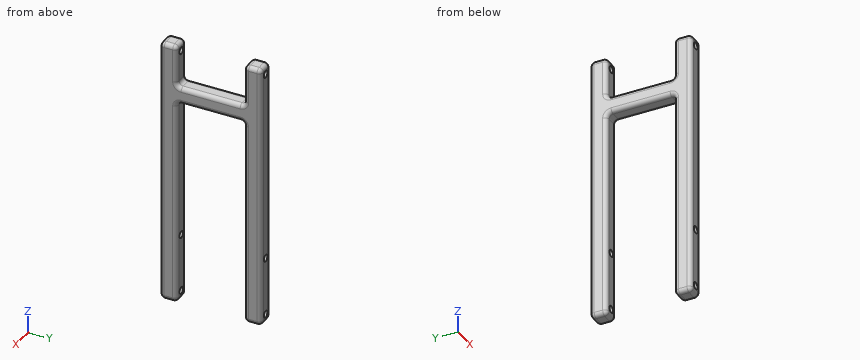
Autodesk Inventor part; units mm, degrees
ref_plane "YZ Plane" through (0, 0, 0) normal (1, 0, 0) x (0, 1, 0)
ref_plane "XZ Plane" through (0, 0, 0) normal (0, 1, 0) x (-1, 0, 0)
ref_plane "XY Plane" through (0, 0, 0) normal (0, 0, 1) x (1, 0, 0)
sketch "Sketch1" plane through (0, 0, 0) normal (0, 1, 0) x (-1, 0, 0)
  line L0 (0, 0) -> (12.7, 0)
  line L1 (12.7, 0) -> (12.7, 203.2)
  line L2 (12.7, 203.2) -> (0, 203.2)
  line L3 (0, 203.2) -> (0, 0)
  circle A0 centre (6.35, 6.35) radius 2.5797
  circle A1 centre (6.35, 196.85) radius 2.5797
  circle A2 centre (6.35, 50.8) radius 2.5797
  dimension "d0" = 12.7
  dimension "d1" = 203.2
  dimension "d2" = 6.35
  dimension "d3" = 6.35
  dimension "d4" = 5.1594
  dimension "d5" = 6.35
  dimension "d6" = 5.1594
  dimension "d7" = 6.35
  dimension "d19" = 5.1594
  dimension "d20" = 6.35
  dimension "d21" = 50.8
extrude "Extrusion1" add sketch "Sketch1" along normal blind 76.2
sketch "Sketch2" plane through (0, 0, 203.2) normal (1, 0, 0) x (0, 0, -1)
  line L0 (203.2, 76.2) -> (0, 76.2)
  line L1 (0, 76.2) -> (31.75, 76.2)
  line L2 (31.75, 76.2) -> (31.75, 0)
  line L3 (31.75, 0) -> (0, 0)
  line L4 (0, 0) -> (0, 76.2)
  line L5 (203.2, 76.2) -> (177.8, 76.2)
  line L6 (177.8, 76.2) -> (177.8, 0)
  line L7 (177.8, 0) -> (203.2, 0)
  line L8 (203.2, 0) -> (203.2, 76.2)
  line L9 (203.2, 0) -> (203.2, 76.2)
  line L10 (203.2, 63.5) -> (0, 63.5)
  line L11 (0, 63.5) -> (0, 12.7)
  line L12 (0, 12.7) -> (203.2, 12.7)
  line L13 (203.2, 12.7) -> (203.2, 63.5)
  line L14 (0, 0) -> (203.2, 0)
  line L15 (31.75, 63.5) -> (44.45, 63.5)
  line L16 (44.45, 63.5) -> (44.45, 12.7)
  line L17 (44.45, 12.7) -> (31.75, 12.7)
  line L18 (31.75, 12.7) -> (31.75, 63.5)
  line L19 (177.8, 63.5) -> (165.1, 63.5)
  line L20 (165.1, 12.7) -> (177.8, 12.7)
  line L21 (177.8, 12.7) -> (177.8, 63.5)
  line L22 (139.7, 63.5) -> (139.7, 12.7)
  line L23 (139.7, 63.5) -> (127, 63.5)
  line L24 (127, 63.5) -> (127, 12.7)
  line L25 (127, 12.7) -> (139.7, 12.7)
  line L26 (139.7, 12.7) -> (139.7, 63.5)
  point P0 (177.8, 12.7)
  point P1 (184.15, 63.5)
  point P2 (0, 12.7)
  point P3 (31.75, 12.7)
  point P4 (19.05, 63.5)
  point P5 (0, 63.5)
  point P6 (44.45, 63.5)
  point P7 (31.75, 12.7)
  dimension "d10" = 31.75
  dimension "d12" = 25.4
  dimension "d13" = 76.2
  dimension "d14" = 203.2
  dimension "d15" = 50.8
  dimension "d16" = 12.7
  dimension "d22" = 12.7
  dimension "d24" = 63.5
  dimension "d25" = 12.7
extrude "Extrusion2" cut sketch "Sketch2" against normal blind 12.7 contours L8 L12 L6 L10 | L6 L12 L22 L10 | L2 L12 L4 L10 | L10 L24 L12 L16 | L22 L12 L24 L10
fillet "Fillet1" radius 3.175 36 edges at (0, 38.1, 158.75) (0, 38.1, 171.45) (-12.7, 38.1, 171.45) (-12.7, 38.1, 158.75) (0, 63.5, 79.375) (0, 76.2, 101.6) (-12.7, 76.2, 101.6) (-12.7, 63.5, 79.375) (0, 63.5, 187.325) (-12.7, 63.5, 187.325) (-6.35, 63.5, 158.75) (-6.35, 63.5, 171.45) (-12.7, 12.7, 79.375) (0, 12.7, 79.375) (-12.7, 0, 101.6) (0, 0, 101.6) (0, 12.7, 187.325) (-12.7, 12.7, 187.325) (-6.35, 12.7, 171.45) (-6.35, 12.7, 158.75) (-6.35, 12.7, 203.2) (0, 6.35, 203.2) (-6.35, 0, 203.2) (-12.7, 6.35, 203.2) (0, 6.35, 0) (-6.35, 0, 0) (-12.7, 6.35, 0) (-6.35, 12.7, 0) (-6.35, 76.2, 0) (0, 69.85, 0) (-6.35, 63.5, 0) (-12.7, 69.85, 0) (0, 69.85, 203.2) (-6.35, 63.5, 203.2) (-12.7, 69.85, 203.2) (-6.35, 76.2, 203.2)
properties part number "inner swing"
Geometry: final body of the model. Coordinates: model frame, mm. Give positions to 0.01 mm unless a question says otherwise; leave off trailing zeros. Write each loop counter-clockwise with the first axis right and the second up, starting at its lowest first coordinate (ties: lowest second). Pieces come first, ordered by that corner, then holes. Notation, with made-up numbers: M -37,-15 L -12,-15 A33 cw -12,24 Z; hole C 0,-31.75 d6. An arc over 180 degrees is marked long. Answer in a Markdown table with one row per item. Add a question column.
(1) First-contact query: pin 1 (5 mm diameter, centred on x = -10.5, y = 29, fed in from -Z); pin 2 (6 mm diameter, centred on x = -4, y = 60, fed in from +Z); pin 3 (3 mm diameter, centred on x = -6.5, y = 30, fed in from +Z). Flat tips, straight axial feed; report the tip coordinate or a pass-through.
(2) Section D-D on x = -6.35. State how many separate pieces and enclosed holes the cut face has, and give its area (3 significant figures).
(3) Ray query, line 1 (Z direction, x = -6.35, y = 7.75); line 2 (Y direction, x = -4, z = 126.5); line 3 (X direction, y = 4.5, z = 6.35). Return the intervals inside material, ascending.
(4) Section C-C on z = 32.5. Return loops of the section in (x, y) (3 decimals), and give its area (3 significant figures).
(5) Section A-A on z = 196.85. Return loops of the section in (x, y) (3 decimals), and give its area (3 significant figures).
(6) Section B-B on y = 7.5. Return loops of the section in (x, z) (3 decimals).
Result set:
| question | item | result |
|---|---|---|
| 1 | pin 1 | stops at z = 158.75 |
| 1 | pin 2 | stops at z = 172.91 |
| 1 | pin 3 | stops at z = 171.45 |
| 2 | separate pieces | 7 |
| 2 | enclosed holes | 0 |
| 2 | area | 5,400 mm^2 |
| 3 | line 1 | z = 0 to 3.77, 8.93 to 48.22, 53.38 to 194.27, 199.43 to 203.2 |
| 3 | line 2 | y = 0 to 12.7, 63.5 to 76.2 |
| 3 | line 3 | x = -12.7 to -8.93, -3.77 to 0 |
| 4 | outline | M -12.7,3.175 A3.175 ccw -9.525,0 L -3.175,0 A3.175 ccw 0,3.175 L 0,9.525 A3.175 ccw -3.175,12.7 L -9.525,12.7 A3.175 ccw -12.7,9.525 Z; M -12.7,66.675 A3.175 ccw -9.525,63.5 L -3.175,63.5 A3.175 ccw 0,66.675 L 0,73.025 A3.175 ccw -3.175,76.2 L -9.525,76.2 A3.175 ccw -12.7,73.025 Z |
| 4 | area | 305 mm^2 |
| 5 | outline | M -12.7,3.175 A3.175 ccw -9.525,0 L -8.93,0 L -8.93,12.7 L -9.525,12.7 A3.175 ccw -12.7,9.525 Z; M -12.7,66.675 A3.175 ccw -9.525,63.5 L -8.93,63.5 L -8.93,76.2 L -9.525,76.2 A3.175 ccw -12.7,73.025 Z; M -3.77,0 L -3.175,0 A3.175 ccw 0,3.175 L 0,9.525 A3.175 ccw -3.175,12.7 L -3.77,12.7 Z; M -3.77,63.5 L -3.175,63.5 A3.175 ccw 0,66.675 L 0,73.025 A3.175 ccw -3.175,76.2 L -3.77,76.2 Z |
| 5 | area | 174 mm^2 |
| 6 | outline | M -12.7,3.175 A3.175 ccw -9.525,0 L -3.175,0 A3.175 ccw 0,3.175 L 0,200.025 A3.175 ccw -3.175,203.2 L -9.525,203.2 A3.175 ccw -12.7,200.025 Z; hole C -6.35,6.35 d5.159; hole C -6.35,50.8 d5.159; hole C -6.35,196.85 d5.159 |
